from build123d import *

# Parameters (mm, degrees)
SKETCH1_W           = 66
SKETCH1_H           = 42
BOSS_EXTRUDE1_DEPTH = 12
SKETCH2_W           = 12
SKETCH2_H           = 42
BOSS_EXTRUDE2_DEPTH = 26.995042498
SKETCH4_R           = 21
BOSS_EXTRUDE8_DEPTH = 12
BOSS_EXTRUDE9_DEPTH = 6
CUT_EXTRUDE1_DEPTH  = 12


with BuildPart() as part:
    # Sketch1 → Boss-Extrude1 (new body)
    with BuildSketch(Plane(origin=(0, 0, 0), x_dir=(1, 0, 0), z_dir=(0, 1, 0))):
        Rectangle(SKETCH1_W, SKETCH1_H)
    extrude(amount=BOSS_EXTRUDE1_DEPTH)

    # Sketch2 → Boss-Extrude2 (add)
    with BuildSketch(Plane(origin=(0, 12, 0), x_dir=(1, 0, 0), z_dir=(0, 1, 0))):
        with Locations((-27, 0)):
            Rectangle(SKETCH2_W, SKETCH2_H)
    extrude(amount=BOSS_EXTRUDE2_DEPTH)

    # Sketch4 → Boss-Extrude8 (add)
    with BuildSketch(Plane(origin=(-21, 0, 0), x_dir=(0, 0, -1), z_dir=(1, 0, 0))):
        with Locations((0, 38.995042498)):
            Circle(SKETCH4_R)
    extrude(amount=-BOSS_EXTRUDE8_DEPTH)

    # Sketch8 → Boss-Extrude9 (add, symmetric)
    with BuildSketch(Plane.XY):
        Polygon((-21, 12), (-21, 55.038969321), (33, 12), align=None)
    extrude(amount=BOSS_EXTRUDE9_DEPTH, both=True)

    # Sketch12 → Cut-Extrude1 (cut)
    with BuildSketch(Plane(origin=(0, 12, 0), x_dir=(1, 0, 0), z_dir=(0, 1, 0))):
        Polygon((33, -12.935780303), (33, -21), (23.965356614, -21), align=None)
        Polygon((33, 13.5), (33, 21), (23.455136658, 21), align=None)
    extrude(amount=-CUT_EXTRUDE1_DEPTH, mode=Mode.SUBTRACT)


solid = part.part
Part model, mm, in its own coordinate system. A direction names the side the tool comes from. Coordinates: 2 decimals unless noted, no trailing zeros. Order: outer loops, then holes, each group sorted by start corner. A loop starts at its lowest first (then second) coordinate and runs counter-clockwise, first axis right, second up. Notation, with made-up numbers: M 84,62 L 140,62 A18 ccw 140,80 Z; hole C 37,88 d7. An arc over 180 degrees is marked long. Use a Markdown table: item, result.
(1) Flat gauge pins, fed straight in: pin 1 (4 mm diameter, centred on x = -3, y = 17.5, fed in from -Z); pin 2 (21 mm diameter, centred on y = 42.5, z = 9, fed in from +X); pin 3 (2 mm diameter, centred on x = -18, z = -3.5, fed in from +Y). Where does each tip first touch, or does it go through?
A:
| item | result |
|---|---|
| pin 1 | stops at z = -6 |
| pin 2 | stops at x = 7.36 |
| pin 3 | stops at y = 53.44 |
(2) Tool access for faces 1 (the flat face through (-6, 24, -6)), 2 (the flat face through (-6, 24, 6)), 3 (the flat face through (-21, 36, 10)): list every direction of +Z, -Z, +X, -X, +Y, -Y with a clear straight run to the whole face (end or side of a thin tool).
A:
| item | result |
|---|---|
| face 1 | -Z, +X, +Y |
| face 2 | +Z, +X, +Y |
| face 3 | +X, +Y |
(3) Cut at A-A on z = 0. Write the cut outline in (x, y), then the cut area to 3 significant figures.
A:
| item | result |
|---|---|
| outline | M -33,0 L 33,0 L 33,12 L -21,55.04 L -21,60 L -33,60 Z |
| area | 2,530 mm^2 |
(4) Cut at C-C on y = 53. Write the cut outline in (x, z), then the cut area to 3 significant figures.
A:
| item | result |
|---|---|
| outline | M -33,-15.65 L -21,-15.65 L -21,-6 L -18.44,-6 L -18.44,6 L -21,6 L -21,15.65 L -33,15.65 Z |
| area | 406 mm^2 |
(5) Cut at D-D on z = 4.5. Write the cut outline in (x, y).
A:
| item | result |
|---|---|
| outline | M -33,0 L 33,0 L 33,12 L -21,55.04 L -21,59.51 L -33,59.51 Z |
(6) Probe L1, parallel to Z at x = 8.5, y = 16.5; L2, parallel to Y at x = -10.5, z = 18.5; L3, parallel to X at y = 32, z = -17. List the from-to ranges inside material, lowest first.
A:
| item | result |
|---|---|
| L1 | z = -6 to 6 |
| L2 | y = 0 to 12 |
| L3 | x = -33 to -21 |
(7) Cut at B-B on x = 20.5. Write the cut outline in (y, z), then the cut area to 3 significant figures.
A:
| item | result |
|---|---|
| outline | M 0,-21 L 12,-21 L 12,-6 L 21.96,-6 L 21.96,6 L 12,6 L 12,21 L 0,21 Z |
| area | 624 mm^2 |
